```python
from build123d import *

# Parameters (mm, degrees)
GRUNDK_RPER_DEPTH               = 100
SCHRAEGEN_VORNE_DEPTH           = 100
SCHNITT_LINEAR_AUSTRAGEN4_DEPTH = 45
WANDUNG3_T                      = -1.75
SKIZZE6_R                       = 15
SCHNITT_LINEAR_AUSTRAGEN6_DEPTH = 2


with BuildPart() as part:
    # Skizze1 → Grundkörper (new body)
    with BuildSketch(Plane.XY):
        Polygon((0, 0), (100, 0), (85, 45), (15, 45), align=None)
    extrude(amount=-GRUNDK_RPER_DEPTH)

    # Skizze2 → Schraegen_vorne (cut)
    with BuildSketch(Plane(origin=(0, 0, 0), x_dir=(0, 0, -1), z_dir=(1, 0, 0))):
        Polygon((100, 0), (73.544212344, 45), (100, 45), align=None)
    schraegen_vorne = extrude(amount=SCHRAEGEN_VORNE_DEPTH, mode=Mode.SUBTRACT)

    # Spiegel_Schraege_hinten: Schraegen_vorne across plane
    add(schraegen_vorne.mirror(Plane.XY.offset(-50)), mode=Mode.SUBTRACT)

    # Skizze4 → Schnitt-Linear austragen4 (cut)
    with BuildSketch(Plane.XZ):
        Polygon((100, 0), (75, -40), (25, -40), (0, 0), align=None)
    extrude(amount=-SCHNITT_LINEAR_AUSTRAGEN4_DEPTH, mode=Mode.SUBTRACT)

    # Wandung3
    wandung3_openings = [part.faces().sort_by_distance(p)[0] for p in [
        (50, 0, -63.80952381),
    ]]
    offset(amount=WANDUNG3_T, openings=wandung3_openings, kind=Kind.INTERSECTION)

    # Skizze6 → Schnitt-Linear austragen6 (cut)
    with BuildSketch(Plane.XY.offset(-40)):
        with Locations((50, 20)):
            Circle(SKIZZE6_R)
    extrude(amount=-SCHNITT_LINEAR_AUSTRAGEN6_DEPTH, mode=Mode.SUBTRACT)


solid = part.part
```
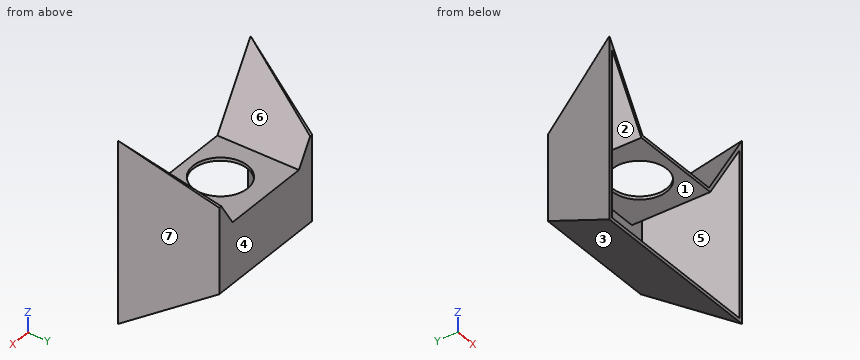
Verification items for the finished model (mm, model axes). Face numbers are marked on the shaded views. A direction names the side the tool comes from. Coordinates: 2 decimals unless noted, no trailing zeros. Order: outer loops, then holes, each group sorted by start corner. A loop starts at its lowest first (then second) coordinate and runs counter-clockwise, first axis right, second up. Notation, with made-up numbers: (66.25, 20) - (111.25, 20) arc R31 cw to (111.25, 48) - close; hole circle Ø5 at (60.25, 37). An arc over 180 degrees is marked (long way). Return JSON: item names as keys, results as strings.
(1) Access from +Z, -Z, +X, -X, +Y, -Y to the whole of each face (thin tool, end or side, straight path). Record for the marked faces 5, 6 and 7.
Filled sheet:
{"face 5": "-Y", "face 6": "+Z, +Y, -Y", "face 7": "+Z, -Z, +X, +Y"}
(2) Section check D-D, the plane x = 87.5. Record the cut outline in (y, z).
Filled sheet:
{"outline": "(0, -100) - (37.5, -77.95) - (37.5, -22.05) - (34.02, -20) - (0, -20) - (0, -23.3) - (31.97, -23.3) - (31.97, -79.18) - (0, -97.97) - close"}
(3) Thickness scan on line 1 along Y through (x, z) = (50, -40.8); line 2 along X through (y, z) = (33, -39) (3 decimals); line 3 along Z through (x, y) = (24, 24). Record the ranges inside material, lowest first.
Filled sheet:
{"line 1": "y = 0 to 5, 35 to 45", "line 2": "x = 11 to 12.845, 22.311 to 24.375, 75.625 to 77.689, 87.155 to 89", "line 3": "z = -85.89 to -83.86, -41.7 to -38.4"}
(4) Section check A-A, the plane x = 54.5. Record the cut outline in (y, z), and give its area (3 significant figures).
Filled sheet:
{"outline": "(0, -100) - (45, -73.54) - (45, -40) - (34.31, -40) - (34.31, -41.75) - (43.25, -41.75) - (43.25, -72.54) - (0, -97.97) - close; (0, -41.75) - (5.69, -41.75) - (5.69, -40) - (0, -40) - close", "area": "173 mm^2"}
(5) Go/stop test with flat-tipped pins: pin 1 (22.5 mm diameter, centred on x = 44.5, y = 12.5, fed in from +Z); pin 2 (3 mm diameter, centred on x = 70, z = -46.5, fed in from -Y); pin 3 (8 mm diameter, centred on y = 10, z = -30.5, fed in from +X). Record where each tip stops, or that it passes through.
Filled sheet:
{"pin 1": "stops at z = -40", "pin 2": "stops at y = 43.25", "pin 3": "stops at x = 98"}
(6) Section check C-C, the plane y = 14. Record the cut outline in (x, z).
Filled sheet:
{"outline": "(4.67, -91.77) - (95.33, -91.77) - (95.33, -8.23) - (94.86, -8.23) - (75, -40) - (63.75, -40) - (63.75, -41.75) - (75.97, -41.75) - (93.49, -13.72) - (93.49, -89.74) - (6.51, -89.74) - (6.51, -13.72) - (24.03, -41.75) - (36.25, -41.75) - (36.25, -40) - (25, -40) - (5.14, -8.23) - (4.67, -8.23) - close"}
(7) Section check B-B, the plane z = -70. Record the cut outline in (x, y).
Filled sheet:
{"outline": "(0, 0) - (1.84, 0) - (16.26, 43.25) - (83.74, 43.25) - (98.16, 0) - (100, 0) - (85, 45) - (15, 45) - close"}
(8) Mould release check, pull along Z, two halves, no side actions. Record for the marked faces 1, 2, 3 and 4: pulls with the +Z half, pulls with the -Z half, needs draft (parallel to the pull), parting line crosses it, or undercut.
Filled sheet:
{"face 1": "undercut", "face 2": "undercut", "face 3": "pulls with the -Z half", "face 4": "needs draft"}
